from build123d import *

# Parameters (mm, degrees)
F1_DEPTH       = 4
F3_D           = 3.3
F3_CBORE_D     = 6.5
F3_CBORE_DEPTH = 3
F5_W           = 6.096
F5_H           = 15.1188707026
F5_H_2         = 6.096
F6_DEPTH       = 2.032
F4_R           = 1.651
F7_DEPTH       = 1.27


with BuildPart() as f1:
    # F0 (on Front) → F1 (new body)
    with BuildSketch(Plane.XZ):
        Polygon((44.45, 74), (-12.7, 74), (-12.7, 49.4), (-22.352, 49.4), (-22.352, 24), (44.45, 24), align=None)
    extrude(amount=F1_DEPTH)

    # F3 (through all)
    with Locations(Plane.XZ.offset(4)):
        with Locations((-11.811, 41), (11.811, 41)):
            CounterBoreHole(F3_D / 2, F3_CBORE_D / 2, F3_CBORE_DEPTH)

    # F5 (on face) → F6 (cut)
    with BuildSketch(Plane(origin=(0, 0, 0), x_dir=(-1, 0, 0), z_dir=(0, 1, 0))):
        with Locations((4.699, 74.6198353513)):
            Rectangle(F5_W, F5_H)
        with Locations((-37.719, 31.7544)):
            Rectangle(F5_W, F5_H_2)
    extrude(amount=-F6_DEPTH, mode=Mode.SUBTRACT)

    # F4 (on face) → F7 (cut)
    with BuildSketch(Plane.XZ.offset(4)):
        with Locations((37.719, 31.7544)):
            Circle(F4_R)
        with Locations((-4.699, 70.1084)):
            Circle(F4_R)
    extrude(amount=-F7_DEPTH, mode=Mode.SUBTRACT)


solid = f1.part
Part model, mm, in its own coordinate system. A direction names the side the tool comes from. Round coordinates to 2 decimals unless told otherwise and drop trailing zeros. Write each loop counter-clockwise with the first axis right and the second up, starting at its lowest first coordinate (ties: lowest second). Pieces come first, ordered by that corner, then holes. Notation, with made-up numbers: (66.5, 2) - (88.5, 2) arc R7 ccw to (88.5, 6) - close; hole circle Ø11 at (-3, 37). An arc over 180 degrees is marked (long way). Use CSV: the item, a comma, the result in double quotes.
Item 1: Tool access for faces 1 (the flat face through (34.671, -1, 32)), 2 (the flat face through (-5, -1, 67.06)), 3 (the flat face through (38, -2.73, 32)): list every direction of +Z, -Z, +X, -X, +Y, -Y with a clear straight run to the whole face (end or side of a thin tool).
Results list:
face 1,"+Y"
face 2,"+Z, +Y"
face 3,"-Y"
Item 2: Slice it at A-A, the plane z = 41. Write the cut outline in (x, y), then the cut area to 3 significant figures.
Results list:
outline,"(-22.35, -4) - (-15.06, -4) - (-15.06, -1) - (-13.46, -1) - (-13.46, 0) - (-22.35, 0) - close; (-10.16, -1) - (-8.56, -1) - (-8.56, -4) - (8.56, -4) - (8.56, -1) - (10.16, -1) - (10.16, 0) - (-10.16, 0) - close; (13.46, -1) - (15.06, -1) - (15.06, -4) - (44.45, -4) - (44.45, 0) - (13.46, 0) - close"
area,"222 mm²"
Item 3: Flat gauge pins, fed straight in: P1, Ø8.5, axis at x = 11.811, z = 41, coming from the -Y side; P2, Ø1, axis at x = 38, z = 32.5, coming from the -Y side; P3, Ø2.5, axis at x = -11.811, z = 41, coming from the +Y side; P4, Ø1.2, axis at y = -3, z = 66, coming from the -X side. Where does each tip first touch, or does it go through?
Results list:
P1,"stops at y = -4"
P2,"stops at y = -2.73"
P3,"passes through"
P4,"stops at x = -12.7"
Item 4: Wall check: L1, parallel to Z at x = 38.5, y = -0.15; L2, parallel to X at y = -0.5, z = 29.5; L3, parallel to X at y = -3.1, z = 41.5. Give the ranges that are in metal, low to high.
Results list:
L1,"z = 24 to 28.71, 34.8 to 74"
L2,"x = -22.35 to 34.67, 40.77 to 44.45"
L3,"x = -22.35 to -15.02, -8.6 to 8.6, 15.02 to 44.45"
Item 5: Pull direction X, two halves, no side cores. Call faces 4 (the cylindrical face through (-12.7, -0.49, 42.39)), 5 (the flat face through (-12.7, -2, 62)), 6 (the flat face through (11, -2, 24)): pulls with the +X half, pulls with the -X half, needs draft (parallel to the pull), parting line crosses it, or undercut.
Results list:
face 4,"undercut"
face 5,"pulls with the -X half"
face 6,"needs draft"
